from build123d import *

# Parameters (mm, degrees)
F0_R     = 50
F1_DEPTH = 18
F2_R     = 5
F3_D     = 5


with BuildPart() as f1:
    # F0 (on Right) → F1 (new body)
    with BuildSketch(Plane.YZ):
        Circle(F0_R)
    extrude(amount=F1_DEPTH)

    # F2
    f2_edges = [f1.edges().sort_by_distance(p)[0] for p in [
        (18, -50, 0),
        (0, -50, 0),
    ]]
    fillet(f2_edges, radius=F2_R)

    # F3 (through all)
    with Locations(Plane(origin=(0, 0, 0), x_dir=(0, 1, 0), z_dir=(-1, 0, 0))):
        with Locations((0, 0)):
            Hole(F3_D / 2)


solid = f1.part
The model under review builds one solid part; all positions refer to its coordinate system, in mm. Round coordinates to 2 decimals unless told otherwise and drop trailing zeros. Loops run counter-clockwise (first coordinate to the right, second up) from the corner with the lowest first, then second, coordinate; pieces in that order, holes last. Notation, with made-up numbers: (46, 35.5) -> (100, 35.5) arc R27 ccw to (100, 53.5) -> close; hole circle Ø8 at (23.5, 70.5). An arc over 180 degrees is marked (long way). Write item = value, one per line. Start each with the question number.
Item 1: Mouldability with a two-part tool opening along Z and no side actions: class faces 1 (the cylindrical face through (9.13, 0.54, 2.44)), 2 (the cylindrical face through (8.94, 47.69, 15.02)), 3 (the flat face through (0, -1, -9)) as released by +Z, released by -Z, zero draft, split by the parting line, or undercut.
Item 2: To check wall thickness, follow L1, parallel to Z at x = 9.25, y = 0; L2, parallel to Y at x = 11.25, z = 39; L3, parallel to Z at x = 10.75, y = 9. State the ranges of each line that lie inside material, in increasing order.
Item 3: Take a section at D-D on x = 14.75. Give the boundary of the cut face in (y, z), plus the area to 3 significant figures.
Item 4: Take a section at A-A on z = 0. Give the boundary of the cut face in (x, y), plus the area to 3 significant figures.
Item 5: Take a section at C-C on x = 7.75. Give the boundary of the cut face in (y, z), plus the area to 3 significant figures.
Item 6: Insertion check: pin 1 (1.5 mm diameter, centred on x = 5.5, z = -39, fed in from -Y); pin 2 (3 mm diameter, centred on x = 2, y = -20.5, fed in from +Z); pin 3 (1 mm diameter, centred on x = 12.5, z = 8.5, fed in from +Y). Each pin has a flat end and moves straight along its axis. Give the tip position at first contact, or say it passes through.
Result:
q1.face_1 = undercut
q1.face_2 = split by the parting line
q1.face_3 = zero draft
q2.L1 = -50 to -2.5, 2.5 to 50
q2.L2 = -31.29 to 31.29
q2.L3 = -49.18 to 49.18
q3.outline = circle Ø99.37 at (0, 0); hole circle Ø5 at (0, 0)
q3.area = 7,740 mm²
q4.outline = (0, -45) arc R5 ccw to (5, -50) -> (13, -50) arc R5 ccw to (18, -45) -> (18, -2.5) -> (0, -2.5) -> close; (0, 2.5) -> (18, 2.5) -> (18, 45) arc R5 ccw to (13, 50) -> (5, 50) arc R5 ccw to (0, 45) -> close
q4.area = 1,690 mm²
q5.outline = circle Ø100 at (0, 0); hole circle Ø5 at (0, 0)
q5.area = 7,830 mm²
q6.pin_1 = -32.2
q6.pin_2 = 45.64
q6.pin_3 = 49.36
